Input: dimensioned drawing with shaded views. Units: mm. Origin: part minimum x, y, z. A direction names the side the tool comes from. Round coordinates to 2 decimals unless told otherwise and drop trailing zeros. Loops run counter-clockwise (first coordinate to the right, second up) from the corner with the lowest first, then second, coordinate; pieces in that order, holes last. Notation, with made-up numbers: M 26.5,49.25 L 55.5,49.25 A13 ccw 55.5,74.25 Z; hole C -13,88 d11. An arc over 180 degrees is marked long. Answer as a JSON object with one key per item and string values.
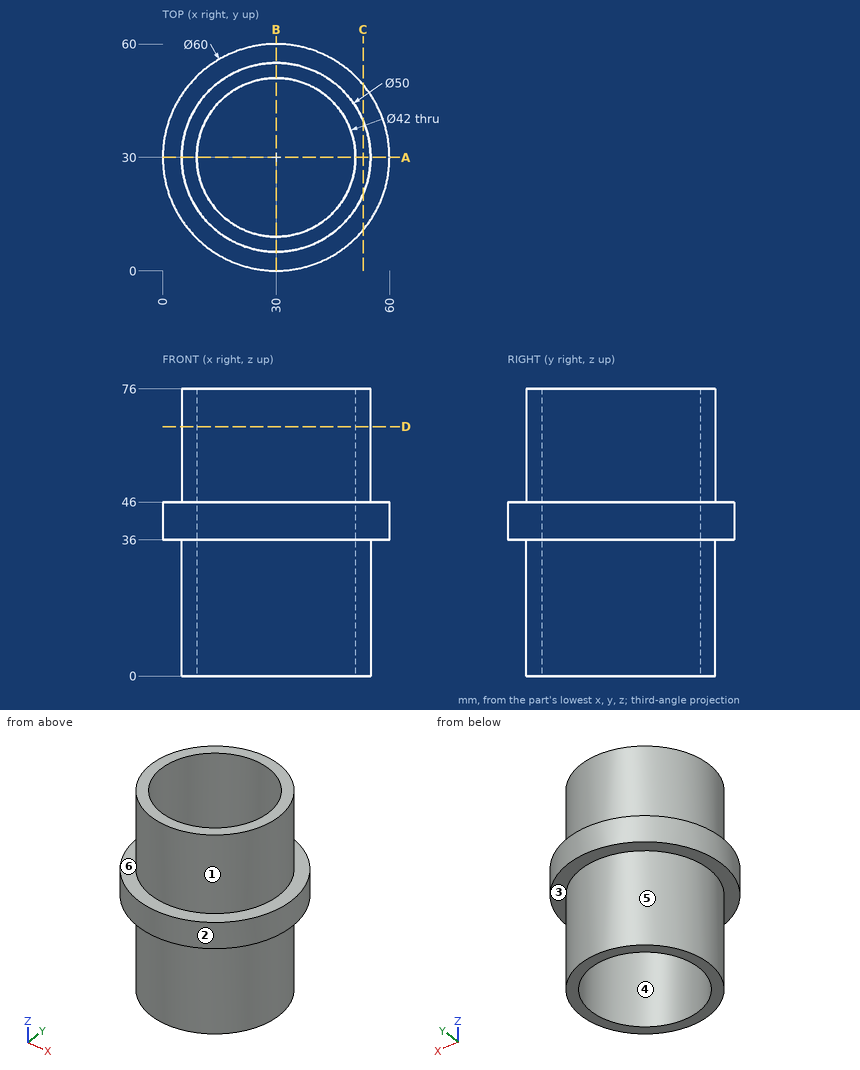
Item 1: Section D-D on z = 66. Return the cut outline in (x, y).
Answer sheet:
{"outline": "C 30,30 d50; hole C 30,30 d42"}
Item 2: Line query: probe 1 along X at (y, z) = (30, 23); probe 2 along Z at (x, y) = (56, 32). Output: solid intervals per line, ascending. Write a range as from..to.
Answer sheet:
{"probe 1": "x = 5..9, 51..55", "probe 2": "z = 36..46"}
Item 3: Pull-direction query (X, two-part tool) for the marked faces 4, 5 and 6; classes: pulls with the +X half, pulls with the -X half, needs draft (parallel to the pull), parting line crosses it, or undercut.
Answer sheet:
{"face 4": "undercut", "face 5": "parting line crosses it", "face 6": "needs draft"}
Item 4: Section C-C on x = 53. Return the cut outline in (y, z).
Answer sheet:
{"outline": "M 10.74,36 L 20.2,36 L 20.2,0 L 39.8,0 L 39.8,36 L 49.26,36 L 49.26,46 L 39.8,46 L 39.8,76 L 20.2,76 L 20.2,46 L 10.74,46 Z"}
Item 5: Access query for the marked faces 1, 2 and 3. Directions: +Z, -Z, +X, -X, +Y, -Y. A direction counts if a zero-diameter tool reaches every point of the face in a straight line with its end or side. Return the directions, or none.
Answer sheet:
{"face 1": "+Z", "face 2": "+Z, -Z", "face 3": "-Z"}
Item 6: Contact query for flat-ended pins moving along their axis: pin 1 Ø1.5 at (y, z) = (53.5, 23) entering from +X; pin 2 Ø4 at (x, y) = (8, 51.5) entering from +Z; pin 3 Ø5 at (x, z) = (44, 58.5) entering from -Y. Output: stop coordinate, or through.
Answer sheet:
{"pin 1": "stops at x = 40.37", "pin 2": "stops at z = 46", "pin 3": "stops at y = 7.8"}
Item 7: Section A-A on y = 30. Return the cut outline in (x, z).
Answer sheet:
{"outline": "M 0,36 L 5,36 L 5,0 L 9,0 L 9,76 L 5,76 L 5,46 L 0,46 Z; M 51,0 L 55,0 L 55,36 L 60,36 L 60,46 L 55,46 L 55,76 L 51,76 Z"}
